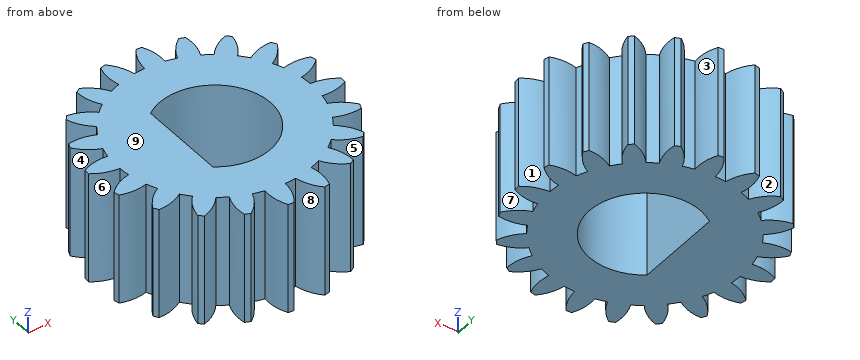
```python
from build123d import *

# Parameters (mm, degrees)
BOSS_EXTRUDE1_DEPTH = 6.35


with BuildPart() as part:
    # Sketch1 → Boss-Extrude1 (new body)
    with BuildSketch(Plane.XY):
        with BuildLine():
            ThreePointArc((5.8600974, 3.801247619), (5.096802915, 3.692613372), (4.401264234, 3.359978717))
            ThreePointArc((4.401264234, 3.359978717), (4.201500823, 3.606656994), (3.987930607, 3.841483218))
            ThreePointArc((3.987930607, 3.841483218), (4.422090523, 4.478605685), (4.645099136, 5.216634837))
            ThreePointArc((4.645099136, 5.216634837), (4.523078796, 5.32277965), (4.398633704, 5.426071004))
            ThreePointArc((4.398633704, 5.426071004), (3.706267339, 5.086882728), (3.147560505, 4.555595099))
            ThreePointArc((3.147560505, 4.555595099), (2.881346432, 4.728469793), (2.605663792, 4.885805977))
            ThreePointArc((2.605663792, 4.885805977), (2.82169274, 5.625908243), (2.805722984, 6.396729128))
            ThreePointArc((2.805722984, 6.396729128), (2.656874194, 6.459972486), (2.506601094, 6.519752753))
            ThreePointArc((2.506601094, 6.519752753), (1.952936493, 5.983212559), (1.585751624, 5.305278091))
            ThreePointArc((1.585751624, 5.305278091), (1.279145776, 5.387427022), (0.968336451, 5.451872005))
            ThreePointArc((0.968336451, 5.451872005), (0.945088011, 6.222507704), (0.691703118, 6.950667004))
            ThreePointArc((0.691703118, 6.950667004), (0.530596234, 6.964818206), (0.369204905, 6.975235676))
            ThreePointArc((0.369204905, 6.975235676), (0.008438615, 6.293863858), (-0.131281675, 5.5356435))
            ThreePointArc((-0.131281675, 5.5356435), (-0.44826658, 5.519025359), (-0.763778409, 5.484270816))
            ThreePointArc((-0.763778409, 5.484270816), (-1.024028517, 6.210004756), (-1.490025469, 6.824225165))
            ThreePointArc((-1.490025469, 6.824225165), (-1.647620183, 6.787898993), (-1.804331633, 6.747933933))
            ThreePointArc((-1.804331633, 6.747933933), (-1.936885292, 5.98842791), (-1.835464209, 5.224141554))
            ThreePointArc((-1.835464209, 5.224141554), (-2.13179948, 5.11038304), (-2.421129317, 4.979830988))
            ThreePointArc((-2.421129317, 4.979830988), (-2.892905998, 5.589623275), (-3.525899981, 6.02978062))
            ThreePointArc((-3.525899981, 6.02978062), (-3.664556056, 5.946532932), (-3.801247619, 5.8600974))
            ThreePointArc((-3.801247619, 5.8600974), (-3.692613372, 5.096802915), (-3.359978717, 4.401264234))
            ThreePointArc((-3.359978717, 4.401264234), (-3.606656994, 4.201500823), (-3.841483218, 3.987930607))
            ThreePointArc((-3.841483218, 3.987930607), (-4.478605685, 4.422090523), (-5.216634837, 4.645099136))
            ThreePointArc((-5.216634837, 4.645099136), (-5.32277965, 4.523078796), (-5.426071004, 4.398633704))
            ThreePointArc((-5.426071004, 4.398633704), (-5.086882728, 3.706267339), (-4.555595099, 3.147560505))
            ThreePointArc((-4.555595099, 3.147560505), (-4.728469793, 2.881346432), (-4.885805977, 2.605663792))
            ThreePointArc((-4.885805977, 2.605663792), (-5.625908243, 2.82169274), (-6.396729128, 2.805722984))
            ThreePointArc((-6.396729128, 2.805722984), (-6.459972486, 2.656874194), (-6.519752753, 2.506601094))
            ThreePointArc((-6.519752753, 2.506601094), (-5.983212559, 1.952936493), (-5.305278091, 1.585751624))
            ThreePointArc((-5.305278091, 1.585751624), (-5.387427022, 1.279145776), (-5.451872005, 0.968336451))
            ThreePointArc((-5.451872005, 0.968336451), (-6.222507704, 0.945088011), (-6.950667004, 0.691703118))
            ThreePointArc((-6.950667004, 0.691703118), (-6.964818206, 0.530596234), (-6.975235676, 0.369204905))
            ThreePointArc((-6.975235676, 0.369204905), (-6.293863858, 0.008438615), (-5.5356435, -0.131281675))
            ThreePointArc((-5.5356435, -0.131281675), (-5.519025359, -0.44826658), (-5.484270816, -0.763778409))
            ThreePointArc((-5.484270816, -0.763778409), (-6.210004756, -1.024028517), (-6.824225165, -1.490025469))
            ThreePointArc((-6.824225165, -1.490025469), (-6.787898993, -1.647620183), (-6.747933933, -1.804331633))
            ThreePointArc((-6.747933933, -1.804331633), (-5.98842791, -1.936885292), (-5.224141554, -1.835464209))
            ThreePointArc((-5.224141554, -1.835464209), (-5.11038304, -2.13179948), (-4.979830988, -2.421129317))
            ThreePointArc((-4.979830988, -2.421129317), (-5.589623275, -2.892905998), (-6.02978062, -3.525899981))
            ThreePointArc((-6.02978062, -3.525899981), (-5.946532932, -3.664556056), (-5.8600974, -3.801247619))
            ThreePointArc((-5.8600974, -3.801247619), (-5.096802915, -3.692613372), (-4.401264234, -3.359978717))
            ThreePointArc((-4.401264234, -3.359978717), (-4.201500823, -3.606656994), (-3.987930607, -3.841483218))
            ThreePointArc((-3.987930607, -3.841483218), (-4.422090523, -4.478605685), (-4.645099136, -5.216634837))
            ThreePointArc((-4.645099136, -5.216634837), (-4.523078796, -5.32277965), (-4.398633704, -5.426071004))
            ThreePointArc((-4.398633704, -5.426071004), (-3.706267339, -5.086882728), (-3.147560505, -4.555595099))
            ThreePointArc((-3.147560505, -4.555595099), (-2.881346432, -4.728469793), (-2.605663792, -4.885805977))
            ThreePointArc((-2.605663792, -4.885805977), (-2.82169274, -5.625908243), (-2.805722984, -6.396729128))
            ThreePointArc((-2.805722984, -6.396729128), (-2.656874194, -6.459972486), (-2.506601094, -6.519752753))
            ThreePointArc((-2.506601094, -6.519752753), (-1.952936493, -5.983212559), (-1.585751624, -5.305278091))
            ThreePointArc((-1.585751624, -5.305278091), (-1.279145776, -5.387427022), (-0.968336451, -5.451872005))
            ThreePointArc((-0.968336451, -5.451872005), (-0.945088011, -6.222507704), (-0.691703118, -6.950667004))
            ThreePointArc((-0.691703118, -6.950667004), (-0.530596234, -6.964818206), (-0.369204905, -6.975235676))
            ThreePointArc((-0.369204905, -6.975235676), (-0.008438615, -6.293863858), (0.131281675, -5.5356435))
            ThreePointArc((0.131281675, -5.5356435), (0.44826658, -5.519025359), (0.763778409, -5.484270816))
            ThreePointArc((0.763778409, -5.484270816), (1.024028517, -6.210004756), (1.490025469, -6.824225165))
            ThreePointArc((1.490025469, -6.824225165), (1.647620183, -6.787898993), (1.804331633, -6.747933933))
            ThreePointArc((1.804331633, -6.747933933), (1.936885292, -5.98842791), (1.835464209, -5.224141554))
            ThreePointArc((1.835464209, -5.224141554), (2.13179948, -5.11038304), (2.421129317, -4.979830988))
            ThreePointArc((2.421129317, -4.979830988), (2.892905998, -5.589623275), (3.525899981, -6.02978062))
            ThreePointArc((3.525899981, -6.02978062), (3.664556056, -5.946532932), (3.801247619, -5.8600974))
            ThreePointArc((3.801247619, -5.8600974), (3.692613372, -5.096802915), (3.359978717, -4.401264234))
            ThreePointArc((3.359978717, -4.401264234), (3.606656994, -4.201500823), (3.841483218, -3.987930607))
            ThreePointArc((3.841483218, -3.987930607), (4.478605685, -4.422090523), (5.216634837, -4.645099136))
            ThreePointArc((5.216634837, -4.645099136), (5.32277965, -4.523078796), (5.426071004, -4.398633704))
            ThreePointArc((5.426071004, -4.398633704), (5.086882728, -3.706267339), (4.555595099, -3.147560505))
            ThreePointArc((4.555595099, -3.147560505), (4.728469793, -2.881346432), (4.885805977, -2.605663792))
            ThreePointArc((4.885805977, -2.605663792), (5.625908243, -2.82169274), (6.396729128, -2.805722984))
            ThreePointArc((6.396729128, -2.805722984), (6.459972486, -2.656874194), (6.519752753, -2.506601094))
            ThreePointArc((6.519752753, -2.506601094), (5.983212559, -1.952936493), (5.305278091, -1.585751624))
            ThreePointArc((5.305278091, -1.585751624), (5.387427022, -1.279145776), (5.451872005, -0.968336451))
            ThreePointArc((5.451872005, -0.968336451), (6.222507704, -0.945088011), (6.950667004, -0.691703118))
            ThreePointArc((6.950667004, -0.691703118), (6.964818206, -0.530596234), (6.975235676, -0.369204905))
            ThreePointArc((6.975235676, -0.369204905), (6.293863858, -0.008438615), (5.5356435, 0.131281675))
            ThreePointArc((5.5356435, 0.131281675), (5.519025359, 0.44826658), (5.484270816, 0.763778409))
            ThreePointArc((5.484270816, 0.763778409), (6.210004756, 1.024028517), (6.824225165, 1.490025469))
            ThreePointArc((6.824225165, 1.490025469), (6.787898993, 1.647620183), (6.747933933, 1.804331633))
            ThreePointArc((6.747933933, 1.804331633), (5.98842791, 1.936885292), (5.224141554, 1.835464209))
            ThreePointArc((5.224141554, 1.835464209), (5.11038304, 2.13179948), (4.979830988, 2.421129317))
            ThreePointArc((4.979830988, 2.421129317), (5.589623275, 2.892905998), (6.02978062, 3.525899981))
            ThreePointArc((6.02978062, 3.525899981), (5.946532932, 3.664556056), (5.8600974, 3.801247619))
        make_face()
        with BuildLine():
            Line((-1.905, 2.54), (-1.905, -2.54))
            ThreePointArc((-1.905, -2.54), (3.175, 0), (-1.905, 2.54))
        make_face(mode=Mode.SUBTRACT)
    extrude(amount=BOSS_EXTRUDE1_DEPTH)


solid = part.part
```
Verification items for the finished model (mm, model axes). Face numbers are marked on the shaded views. A direction names the side the tool comes from. Round coordinates to 2 decimals unless told otherwise and drop trailing zeros.
1. Scan lines: L1, parallel to Y at x = -4.25, z = 1.5; L2, parallel to X at y = -1.75, z = 5 (3 decimals); L3, parallel to X at y = 0.5, z = 4.75 (3 decimals). Record each from-to range of solid material in increasing order.
2. Draft check along X on the marked faces 6, 7, 8 and 9. Enter one of: +X half, -X half, draft (parallel to the pull), parting line (faces both ways), or undercut.
3. Access from +Z, -Z, +X, -X, +Y, -Y to the whole of each face (thin tool, end or side, straight path). Record for the marked faces 1, 2, 3, 4 and 5.
4. Gauge pin test, flat ends, axial feed: P1, Ø2, axis at y = -4, z = 1, coming from the +X side; P2, Ø1.5, axis at x = 2.5, z = 3, coming from the +Y side. Record the tip position at first contact, or that the pin passes through.
Answer:
1. L1: y = -5.37 to -4.17, -3.55 to 4.3
1. L2: x = -6.762 to -1.905, 2.649 to 5.67
1. L3: x = -6.967 to -1.905, 3.135 to 5.515
2. face 6: -X half
2. face 7: +X half
2. face 8: undercut
2. face 9: draft
3. face 1: +Z, -Z, +X
3. face 2: +Z, -Z, +Y
3. face 3: +Z, -Z
3. face 4: +Z, -Z, -X
3. face 5: +Z, -Z, -Y
4. P1: stops at x = 5.43
4. P2: stops at y = 6.52
